Model file for the job. Use its own axes, mm. A direction names the side the tool comes from. Coordinates: 2 decimals unless noted, no trailing zeros. Order: outer loops, then holes, each group sorted by start corner. A loop starts at its lowest first (then second) coordinate and runs counter-clockwise, first axis right, second up. Notation, with made-up numbers: M 62.25,85.25 L 95.25,85.25 A18 cw 95.25,118.25 Z; hole C -10.5,86.5 d7. An arc over 180 degrees is marked long. Return JSON: item names as keys, results as strings.
```python
from build123d import *

# Parameters (mm, degrees)
SKETCH1_R                = 5
BOSS_EXTRUDE1_DEPTH      = 15
BOSS_EXTRUDE3_DEPTH      = 5
BOSS_EXTRUDE3_DEPTH_BACK = 20
SKETCH4_R                = 5
FILLET1_R                = 5


with BuildPart() as part:
    # Sketch1 → Boss-Extrude1 (new body)
    with BuildSketch(Plane(origin=(0, 0, 0), x_dir=(0, 0, -1), z_dir=(1, 0, 0))):
        with BuildLine():
            Line((-201.009068176, 7.568692759), (100, 7.5))
            ThreePointArc((100, 7.5), (107.48293277, -0.50568484), (98.990931823, -7.431808758))
            Line((98.990931823, -7.431808758), (-201.009068176, -7.431307241))
            Line((-201.009068176, -7.431307241), (-201.009068176, 7.568692759))
        make_face()
        with Locations((100, 0)):
            Circle(SKETCH1_R, mode=Mode.SUBTRACT)
    extrude(amount=BOSS_EXTRUDE1_DEPTH)

    # Sketch4 → Boss-Extrude3 (add, two sides: drawn at the far end of the back side and taken through both)
    with BuildSketch(Plane(origin=(15, 0, 0), x_dir=(0, 0, -1), z_dir=(1, 0, 0)).offset(-BOSS_EXTRUDE3_DEPTH_BACK)):
        with Locations((-193.509068176, 0.066981001)):
            Circle(SKETCH4_R)
    extrude(amount=BOSS_EXTRUDE3_DEPTH + BOSS_EXTRUDE3_DEPTH_BACK)

    # Fillet1
    fillet1_edges = [part.edges().sort_by_distance(p)[0] for p in [
        (7.5, 7.568692759, 201.009068176),
        (7.5, -7.431307241, 201.009068176),
    ]]
    fillet(fillet1_edges, radius=FILLET1_R)


solid = part.part
```
Item 1: Saw through at A-A (x = 10). Write the cut outline in (y, z), and give its area (3 significant figures).
Check result:
{"outline": "M -7.43,-98.99 A7.5 ccw long 7.5,-100 L 7.57,196.01 A5 ccw 2.57,201.01 L -2.43,201.01 A5 ccw -7.43,196.01 Z; hole C 0,-100 d10", "area": "4,500 mm2"}
Item 2: Saw through at C-C (z = -43.5). Write the cut outline in (x, y), and give its area (3 significant figures).
Check result:
{"outline": "M 0,-7.43 L 15,-7.43 L 15,7.51 L 0,7.51 Z", "area": "224 mm2"}
Item 3: Saw through at B-B (z = 53.5). Write the cut outline in (x, y), and give its area (3 significant figures).
Check result:
{"outline": "M 0,-7.43 L 15,-7.43 L 15,7.54 L 0,7.54 Z", "area": "224 mm2"}
Item 4: Drop flat-ended pins along their axis: pin 1 Ø2 at (y, z) = (2, 44.5) entering from +X; pin 2 Ø4.5 at (y, z) = (3.5, 37.5) entering from -X; pin 3 Ø5 at (x, y) = (10.5, 6) entering from +Z. Give the stop position or say it passes through.
Check result:
{"pin 1": "stops at x = 15", "pin 2": "stops at x = 0", "pin 3": "stops at z = 200.92"}
Item 5: 3-axis set-ups, long thin cutter, end or side, ignore diameter. For faces 4 (the flat face through (-5, 0, 194)), 5 (the cylindrical face through (17.46, 1.57, 188.74)): which of +Z, -Z, +X, -X, +Y, -Y reach the whole face in a straight line?
Check result:
{"face 4": "+Z, -Z, -X, +Y, -Y", "face 5": "+X"}
Item 6: Wall check: line 1 (Y direction, x = 10.5, z = -100); line 2 (X direction, y = -2.75, z = -42.5); line 3 (Y direction, x = 8.75, z = -77.5). Give the ranges that are in metal, low to high.
Check result:
{"line 1": "y = -7.5 to -5, 5 to 7.5", "line 2": "x = 0 to 15", "line 3": "y = -7.43 to 7.51"}
Item 7: Pull direction Y, two halves, no side cores. Call faces 1 (the cylindrical face through (7.395, -1.915, -104.619)), 2 (the cylindrical face through (-2.54, 1.57, 188.74)), 3 (the flat face through (20, 0, 194)): +Y half, -Y half, draft (parallel to the pull), parting line (faces both ways), or undercut.
Check result:
{"face 1": "undercut", "face 2": "parting line", "face 3": "draft"}
